Autodesk Inventor part; units mm, degrees
ref_plane "YZ Plane" through (0, 0, 0) normal (1, 0, 0) x (0, 1, 0)
ref_plane "XZ Plane" through (0, 0, 0) normal (0, 1, 0) x (-1, 0, 0)
ref_plane "XY Plane" through (0, 0, 0) normal (0, 0, 1) x (1, 0, 0)
ref_plane "Work Plane1" through (0, 0, 0) normal (0, 0, 1) x (1, 0, 0)
sketch "Sketch1" plane through (0, 0, 0) normal (0, 0, 1) x (1, 0, 0)
  line L0 (100, -28) -> (-900, -28)
  line L1 (-439.1083, -28) -> (-403.2461, -28)
  line L2 (-403.2461, -28) -> (-403.2461, 37.4845)
  line L3 (-403.2461, 37.4845) -> (-439.1083, 37.4845)
  line L4 (-439.1083, 37.4845) -> (-439.1083, -28)
  point P0 (0, 0)
extrude "Extrusion1" add sketch "Sketch1" along normal blind 4
fillet "Fillet1" radius 2 4 edges at (-439.1083, -28, 2) (-403.2461, -28, 2) (-439.1083, 37.4845, 2) (-403.2461, 37.4845, 2)
sketch "Sketch2" plane through (0, 0, 4) normal (0, 0, 1) x (1, 0, 0)
  line L0 (100, -17.1) -> (-900, -17.1)
  line L1 (100, -8.9) -> (100, -17.1)
  line L2 (100, -8.9) -> (-900, -8.9)
  line L3 (-900, -17.1) -> (-900, -8.9)
  line L4 (-900, -13) -> (100, -13) construction
  line L5 (-437.1083, -28) -> (-405.2461, -28) construction
  line L6 (-421.1772, -28) -> (-421.1772, 37.4845) construction
  line L7 (-405.2461, 37.4845) -> (-437.1083, 37.4845) construction
  circle A0 centre (-433.1083, -13) radius 3.1
  line L8 (-439.1083, 35.4845) -> (-439.1083, -26) construction
  circle A1 centre (-409.2461, -13) radius 3.1
  point P0 (0, 0)
  dimension "d3" = 6.2
  dimension "d4" = 6
extrude "Extrusion2" cut sketch "Sketch2" against normal through all contours A0 | A1
sketch "Sketch3" plane through (0, 0, 4) normal (0, 0, 1) x (1, 0, 0)
  line L0 (-438.583, 11.7754) -> (-438.5811, 14.7754)
  arc A0 (-438.583, 11.7754) -> (-436.5842, 9.7741) centre (-436.583, 11.7741) ccw
  line L1 (-433.5842, 9.7722) -> (-436.5842, 9.7741)
  line L2 (-433.5823, 12.7722) -> (-433.5842, 9.7722)
  arc A1 (-433.5823, 12.7722) -> (-435.5811, 14.7735) centre (-435.5823, 12.7735) ccw
  line L3 (-438.5811, 14.7754) -> (-435.5811, 14.7735)
  line L4 (-437.6826, 12.2748) -> (-437.6822, 13.0248)
  arc A2 (-434.4822, 13.0228) -> (-437.6822, 13.0248) centre (-436.0822, 13.0238) ccw
  line L5 (-434.4822, 13.0228) -> (-434.4827, 12.2728)
  arc A3 (-437.6826, 12.2748) -> (-434.4827, 12.2728) centre (-436.0827, 12.2738) ccw
  line L6 (-423.4684, 34.7658) -> (-423.4703, 31.7658)
  arc A4 (-423.4684, 34.7658) -> (-425.4671, 36.7671) centre (-425.4684, 34.7671) ccw
  line L7 (-428.4671, 36.769) -> (-425.4671, 36.7671)
  line L8 (-428.469, 33.769) -> (-428.4671, 36.769)
  arc A5 (-428.469, 33.769) -> (-426.4703, 31.7677) centre (-426.469, 33.7677) ccw
  line L9 (-423.4703, 31.7658) -> (-426.4703, 31.7677)
  circle A6 centre (-425.9687, 34.2674) radius 1.6
  point P0 (0, 0)
extrude "Extrusion3" cut sketch "Sketch3" against normal through all contours L4 A2 L5 A3 | A6
sketch "Sketch4" plane through (0, 0, 4) normal (0, 0, 1) x (1, 0, 0)
  line L0 (-394.0939, 43.6118) -> (-422.77, 43.6118)
  line L1 (-422.77, 43.6118) -> (-422.77, 2.3518)
  line L2 (-422.77, 2.3518) -> (-394.0939, 2.3518)
  line L3 (-394.0939, 2.3518) -> (-394.0939, 43.6118)
  point P0 (0, 0)
extrude "Extrusion4" cut sketch "Sketch4" against normal through all
fillet "Fillet2" radius 2 3 edges at (-403.2461, 2.3518, 2) (-422.77, 37.4845, 2) (-422.77, 2.3518, 2)
properties part number "Z limit switch holder"
The model under review builds one solid part; all positions refer to its coordinate system, in mm. A direction names the side the tool comes from. Coordinates: 2 decimals unless noted, no trailing zeros. Loops run counter-clockwise (first coordinate to the right, second up) from the corner with the lowest first, then second, coordinate; pieces in that order, holes last. Notation, with made-up numbers: (-37.75, 61.25) -> (-5.75, 61.25) arc R30 ccw to (-5.75, 100.25) -> close; hole circle Ø2 at (30, -16). An arc over 180 degrees is marked (long way). Answer as CSV lines item,"result".
Item 1: Take a section at A-A, the plane y = -13. State the section outline as (x, z) points.
Results below:
outline,"(-439.11, 0) -> (-436.21, 0) -> (-436.21, 4) -> (-439.11, 4) -> close; (-430.01, 0) -> (-412.35, 0) -> (-412.35, 4) -> (-430.01, 4) -> close; (-406.15, 0) -> (-403.25, 0) -> (-403.25, 4) -> (-406.15, 4) -> close"
Item 2: Draft analysis for pull direction Y (two halves, no side actions). For faces 1 (the flat face through (-425, -2, 0)), 2 (the cylindrical face through (-436.119, 10.674, 2.028)), 3 (the cylindrical face through (-403.85, -27.43, 2.03)), state which applies: +Y half, -Y half, draft (parallel to the pull), parting line (faces both ways), or undercut.
Results below:
face 1,"draft"
face 2,"undercut"
face 3,"-Y half"
Item 3: Take a section at C-C, the plane y = 25. State the section outline as (x, z) points.
Results below:
outline,"(-439.11, 0) -> (-422.77, 0) -> (-422.77, 4) -> (-439.11, 4) -> close"
Item 4: Take a section at B-B, the plane z = 1.15. State the section outline as (x, y) points.
Results below:
outline,"(-439.11, -26) arc R2 ccw to (-437.11, -28) -> (-405.25, -28) arc R2 ccw to (-403.25, -26) -> (-403.25, 0.35) arc R2 ccw to (-405.25, 2.35) -> (-420.77, 2.35) arc R2 cw to (-422.77, 4.35) -> (-422.77, 35.48) arc R2 ccw to (-424.77, 37.48) -> (-437.11, 37.48) arc R2 ccw to (-439.11, 35.48) -> close; hole (-437.68, 12.27) arc R1.6 ccw to (-434.48, 12.27) -> (-434.48, 13.02) arc R1.6 ccw to (-437.68, 13.02) -> close; hole circle Ø6.2 at (-433.11, -13); hole circle Ø3.2 at (-425.97, 34.27); hole circle Ø6.2 at (-409.25, -13)"
Item 5: Insertion check: pin 1 (2 mm diameter, centred on y = 18.5, z = 1, fed in from +X); pin 2 (2.5 mm diameter, centred on x = -425.97, y = 34.27, fed in from -Z); pin 3 (7 mm diameter, centred on x = -433.11, y = -13, fed in from -Z); pin 4 (1.2 mm diameter, centred on x = -415.5, z = 1, fed in from +Y). Each pin has a flat end and moves straight along its axis. Give the tip position at first contact, or say it passes through.
Results below:
pin 1,"stops at x = -422.77"
pin 2,"passes through"
pin 3,"stops at z = 0"
pin 4,"stops at y = 2.35"
Item 6: For L1, parallel to Y at x = -425, z = 3.75; L2, parallel to Y at x = -418.5, z = 1.1; L3, parallel to X at y = 29.5, z = 2, list the stretches that pass through material, from the lowest coordinate up.
Results below:
L1,"y = -28 to 32.99, 35.54 to 37.48"
L2,"y = -28 to 2.35"
L3,"x = -439.11 to -422.77"
Item 7: Machinability: for faces 4 (the flat face through (-413, 2.352, 2)), 5 (the cylindrical face through (-436.046, 14.623, 2.028)), 6 (the flat face through (-439.108, 5, 2)), which of the approach directions +Z, -Z, +X, -X, +Y, -Y give a long, thin tool a straight path to every point of the face, cutting with its end or side? Answer none if there is none.
Results below:
face 4,"+Z, -Z, +X, +Y"
face 5,"+Z, -Z"
face 6,"+Z, -Z, -X, +Y, -Y"
